The model under review builds one solid part; all positions refer to its coordinate system, in mm. A direction names the side the tool comes from. Give positions to 0.01 mm unless a question says otherwise; leave off trailing zeros. Loops run counter-clockwise (first coordinate to the right, second up) from the corner with the lowest first, then second, coordinate; pieces in that order, holes last. Notation, with made-up numbers: M -9,10.25 L 25,10.25 A14 cw 25,25.25 Z; hole C 43,89 d2. An arc over 180 degrees is marked long. One line per item, written item: value. Start each with the question number.
Q1. To check wall thickness, follow line 1 along X through (y, z) = (9, 1.2); line 2 along Y through (x, z) = (7.5, 2.3); line 3 along X through (y, z) = (2.75, 1.1). State the ranges of each line that lie inside material, in increasing order. Write a range as from..to.
Q2. For pin 1 (1.5 mm diameter, centred on x = 21, y = 1.5, fed in from -Z); pin 2 (0.6 mm diameter, centred on y = 7.5, z = 1.5, fed in from -X); pin 3 (0.5 mm diameter, centred on y = 4.5, z = 1.5, fed in from +X); pin 4 (1.4 mm diameter, centred on x = 18, z = 2, fed in from -Y), all flat-tipped, find the tip position at first contact; note any pin that passes through.
Q3. We need section B-B on z = 2.1. Write out the cut boundary in (x, y), plus the area to 3 significant figures.
Q4. For faces 1 (the face through (25.546, 6, 2)), 2 (the face through (5.48, 6, 2)), 3 (the face through (15, 0.254, 2)), list the 3-axis set-ups (+Z, -Z, +X, -X, +Y, -Y) from which the entire face can be reached by the end or side of a thin tool; tool diameter is ignored.
Q5. We need section A-A on y = 10. Write out the cut boundary in (x, z).
```python
from build123d import *

# Parameters (mm, degrees)
SKETCH1_W           = 25.8
SKETCH1_H           = 12.7
BOSS_EXTRUDE1_DEPTH = 0.762
SKETCH2_W           = 20.066
SKETCH2_H           = 12.192
BOSS_EXTRUDE2_DEPTH = 1.778
CHAMFER1_SIZE       = 0.762
SKETCH3_W           = 2.54
SKETCH3_H           = 6.35
BOSS_EXTRUDE3_DEPTH = 0.762


with BuildPart() as part:
    # Sketch1 → Boss-Extrude1 (new body)
    with BuildSketch(Plane.XY):
        with Locations((12.9, 6.35)):
            Rectangle(SKETCH1_W, SKETCH1_H)
    extrude(amount=BOSS_EXTRUDE1_DEPTH)

    # Sketch2 → Boss-Extrude2 (add)
    with BuildSketch(Plane.XY.offset(0.762)):
        with Locations((15.513, 6.35)):
            Rectangle(SKETCH2_W, SKETCH2_H)
    extrude(amount=BOSS_EXTRUDE2_DEPTH)

    # Chamfer1
    chamfer1_edges = [part.edges().sort_by_distance(p)[0] for p in [
        (5.48, 12.446, 1.651),
        (5.48, 0.254, 1.651),
        (25.546, 0.254, 1.651),
        (25.546, 12.446, 1.651),
    ]]
    chamfer(chamfer1_edges, length=CHAMFER1_SIZE)

    # Sketch3 → Boss-Extrude3 (add)
    with BuildSketch(Plane.XY.offset(0.762)):
        with Locations((1.524, 6.35)):
            Rectangle(SKETCH3_W, SKETCH3_H)
    extrude(amount=BOSS_EXTRUDE3_DEPTH)


solid = part.part
```
Solved:
1. line 1: 0.25..2.79, 5.48..25.55
1. line 2: 0.25..12.45
1. line 3: 5.48..25.55
2. pin 1: z = 0
2. pin 2: x = 0.25
2. pin 3: x = 25.55
2. pin 4: y = 0.25
3. outline: M 5.48,1.02 L 6.24,0.25 L 24.78,0.25 L 25.55,1.02 L 25.55,11.68 L 24.78,12.45 L 6.24,12.45 L 5.48,11.68 Z
3. area: 243 mm2
4. face 1: +Z, +X, +Y, -Y
4. face 2: +Z, +Y, -Y
4. face 3: +Z, +X, -X, -Y
5. outline: M 0,0 L 25.8,0 L 25.8,0.76 L 25.55,0.76 L 25.55,2.54 L 5.48,2.54 L 5.48,0.76 L 0,0.76 Z
